from build123d import *

# Parameters (mm, degrees)
F0_W          = 53
F0_H          = 5.5
F0_W_2        = 49
F0_H_2        = 1.5
F1_DEPTH      = 5
F2_W          = 10
F2_H          = 10
F3_DEPTH      = 2
F5_DEPTH      = 5
F5_DEPTH_BACK = 5
F6_SIZE       = 1
F7_R          = 0.99999
F8_R          = 1
F9_SIZE       = 0.5


# Not quite as in the source:
# - a fillet or chamfer is up to 0.001 mm smaller than in the source, because OpenCascade refuses the exact size


with BuildPart() as f1:
    # F0 (on Top) → F1 (new body, symmetric)
    with BuildSketch(Plane.XY):
        Rectangle(F0_W, F0_H)
        Rectangle(F0_W_2, F0_H_2, mode=Mode.SUBTRACT)
    extrude(amount=F1_DEPTH, both=True)

    # F2 (on face) → F3 (cut, through all)
    with BuildSketch(Plane(origin=(0, 2.75, 0), x_dir=(-1, 0, 0), z_dir=(0, 1, 0))):
        Rectangle(F2_W, F2_H)
    extrude(amount=-F3_DEPTH, mode=Mode.SUBTRACT)

    # F4 (on Top) → F5 (join, two sides)
    with BuildSketch(Plane.XY) as f5_sk:
        Polygon((-13.25, -8), (13.25, -8), (13.25, -2.75), (11.25, -2.75), (11.25, -6), (-11.25, -6), (-11.25, -2.75), (-13.25, -2.75), align=None)
    extrude(amount=F5_DEPTH)
    extrude(f5_sk.sketch, amount=-F5_DEPTH_BACK)

    # F6
    f6_edges = [f1.edges().sort_by_distance(p)[0] for p in [
        (0, -2.75, 5),
        (0, -6, 5),
        (11.25, -4.375, 5),
        (-11.25, -4.375, 5),
    ]]
    chamfer(f6_edges, length=F6_SIZE)

    # F7 (radius 1 in the source; OpenCascade refuses exactly that, so slightly less here)
    f7_edges = [f1.edges().sort_by_distance(p)[0] for p in [
        (-5, 2.75, 0),
        (5, 0.75, 0),
        (5, 2.75, 0),
        (-5, 0.75, 0),
    ]]
    fillet(f7_edges, radius=F7_R)

    # F8
    f8_edges = [f1.edges().sort_by_distance(p)[0] for p in [
        (-13.25, -2.75, 0),
        (-26.5, -2.75, 0),
        (26.5, -2.75, 0),
        (-13.25, -8, 0),
        (26.5, 2.75, 0),
        (13.25, -8, 0),
        (13.25, -2.75, 0),
        (-26.5, 2.75, 0),
    ]]
    fillet(f8_edges, radius=F8_R)

    # F9
    f9_edges = [f1.edges().sort_by_distance(p)[0] for p in [
        (-15.749995, 2.75, -5),
        (-15.749995, 2.75, 5),
    ]]
    chamfer(f9_edges, length=F9_SIZE)


solid = f1.part
Build history of the part. All positions in model axes, mm. A direction names the side the tool comes from. Coordinates: 2 decimals unless noted, no trailing zeros. Order: outer loops, then holes, each group sorted by start corner. A loop starts at its lowest first (then second) coordinate and runs counter-clockwise, first axis right, second up. Notation, with made-up numbers: (78, -25) - (117, -25) arc R17 ccw to (117, -13) - close; hole circle Ø11 at (-29.75, -23.75). An arc over 180 degrees is marked (long way). Write item = value, one per line. Start each with the question number.
1) Saw through at A-A on x = -18.5. Write the cut outline in (y, z).
2) Flat gauge pins, fed straight in: pin 1 Ø4 at (x, z) = (0.5, 0) entering from +Y; pin 2 Ø1 at (y, z) = (-5.5, -0.5) entering from -X; pin 3 Ø2.5 at (y, z) = (-5, -1) entering from +X. Where does each tip first touch, or does it go through?
3) Saw through at B-B on x = 9. Write the cut outline in (y, z).
4) Two-plate mould, pull along Y, no slides. Class faces 6 (the face through (-15, 0.75, 0)), 7 (the face through (25.994, -2.233, -4.809)), 8 (the face through (13.25, -5, 0)): pulls with the +Y half, pulls with the -Y half, needs draft (parallel to the pull), parting line crosses it, or undercut.
5) 3-axis set-ups, long thin cutter, end or side, ignore diameter. For faces 1 (the face through (11.74, -4.34, 4.49)), 2 (the face through (-13.25, -5, 0)), 3 (the face through (12.744, -7.483, -4.809)), 4 (the face through (5.285, 1.051, 0.063)), 5 (the face through (-5.285, 2.449, 0.063)): which of +Z, -Z, +X, -X, +Y, -Y reach the whole face in a straight line?
6) Wall check: line 1 along Y through (x, z) = (-8.5, -3.25); line 2 along Y through (x, z) = (22.5, 2). Give the ranges that are in metal, low to high. Write a range as from..to.
From the geometry:
q1.outline = (-2.75, -4.5) - (-2.25, -5) - (-0.75, -5) - (-0.75, 5) - (-2.25, 5) - (-2.75, 4.5) - close; (0.75, -4.5) - (1.25, -5) - (2.25, -5) - (2.75, -4.5) - (2.75, 4.5) - (2.25, 5) - (1.25, 5) - (0.75, 4.5) - close
q2.pin_1 = -0.75
q2.pin_2 = -13.25
q2.pin_3 = 13.25
q3.outline = (-8, -4.5) - (-7.5, -5) - (-6, -5) - (-6, 4) - (-7, 5) - (-7.5, 5) - (-8, 4.5) - close; (-2.75, -5) - (-0.75, -5) - (-0.75, 5) - (-1.75, 5) - (-2.75, 4) - close; (0.75, -4.5) - (1.25, -5) - (2.25, -5) - (2.75, -4.5) - (2.75, 4.5) - (2.25, 5) - (1.25, 5) - (0.75, 4.5) - close
q4.face_6 = undercut
q4.face_7 = pulls with the -Y half
q4.face_8 = needs draft
q5.face_1 = +Z
q5.face_2 = +Z, -Z, -X, -Y
q5.face_3 = -Z, +X, -Y
q5.face_4 = +Z, -Z
q5.face_5 = +Z, -Z, +Y
q6.line_1 = -8..-6, -2.75..-0.75, 0.75..2.75
q6.line_2 = -2.75..-0.75, 0.75..2.75
